```python
from build123d import *

# Parameters (mm, degrees)
SKETCH1_R           = 2.4
BOSS_EXTRUDE1_DEPTH = 2
SKETCH2_R           = 1.5
BOSS_EXTRUDE2_DEPTH = 5
FILLET1_R           = 0.5
CUT_EXTRUDE1_DEPTH  = 0.5


with BuildPart() as part:
    # Sketch1 → Boss-Extrude1 (new body)
    with BuildSketch(Plane(origin=(0, 0, 0), x_dir=(1, 0, 0), z_dir=(0, 1, 0))):
        with Locations(Location((0, 0, 0), (0, 0, 270))):
            Circle(SKETCH1_R)
    extrude(amount=BOSS_EXTRUDE1_DEPTH)

    # Sketch2 → Boss-Extrude2 (add)
    with BuildSketch(Plane(origin=(0, 2, 0), x_dir=(1, 0, 0), z_dir=(0, 1, 0))):
        with Locations(Location((0, 0, 0), (0, 0, 270))):
            Circle(SKETCH2_R)
    extrude(amount=BOSS_EXTRUDE2_DEPTH)

    # Fillet1
    fillet1_edges = [part.edges().sort_by_distance(p)[0] for p in [
        (0, 0, -2.4),
        (0, 2, -2.4),
    ]]
    fillet(fillet1_edges, radius=FILLET1_R)

    # Sketch3 → Cut-Extrude1 (cut)
    with BuildSketch(Plane.XZ):
        Polygon((0.5, 0.5), (1.5, 0.5), (1.5, -0.5), (0.5, -0.5), (0.5, -1.5), (-0.5, -1.5), (-0.5, -0.5), (-1.5, -0.5), (-1.5, 0.5), (-0.5, 0.5), (-0.5, 1.5), (0.5, 1.5), align=None)
    extrude(amount=-CUT_EXTRUDE1_DEPTH, mode=Mode.SUBTRACT)


solid = part.part
```
Verification items for the finished model (mm, model axes). A direction names the side the tool comes from. Coordinates: 2 decimals unless noted, no trailing zeros. Loops run counter-clockwise (first coordinate to the right, second up) from the corner with the lowest first, then second, coordinate; pieces in that order, holes last. Notation, with made-up numbers: (79, -17.5) -> (124, -17.5) arc R29 ccw to (124, 13.5) -> close; hole circle Ø1 at (55.5, 54). An arc over 180 degrees is marked (long way). Answer in a Markdown table with one row per item.
1) Section check C-C (y = 2.25). Record the cut outline in (x, z).
The answers:
| item | result |
|---|---|
| outline | circle Ø3 at (0, 0) |
2) Draft check along X on faces 3 (the face through (0, 7, 0)), 4 (the face through (0, 0.5, 0)), 5 (the face through (2.024, 0.993, 1.29)). Enter one of: released by +X, released by -X, zero draft, split by the parting line, or undercut.
The answers:
| item | result |
|---|---|
| face 3 | zero draft |
| face 4 | undercut |
| face 5 | split by the parting line |
3) Access from +Z, -Z, +X, -X, +Y, -Y to the whole of each face (thin tool, end or side, straight path). Record for faces 1 (the face through (0.45, 4.46, 1.43)), 2 (the face through (-1, 0, 1)).
The answers:
| item | result |
|---|---|
| face 1 | +Y |
| face 2 | +Z, -Z, +X, -X, -Y |
4) Section check A-A (x = 0). Record the cut outline in (y, z).
The answers:
| item | result |
|---|---|
| outline | (0, -1.9) arc R0.5 ccw to (0.5, -2.4) -> (1.5, -2.4) arc R0.5 ccw to (2, -1.9) -> (2, -1.5) -> (7, -1.5) -> (7, 1.5) -> (2, 1.5) -> (2, 1.9) arc R0.5 ccw to (1.5, 2.4) -> (0.5, 2.4) arc R0.5 ccw to (0, 1.9) -> (0, 1.5) -> (0.5, 1.5) -> (0.5, -1.5) -> (0, -1.5) -> close |
5) Scan lines: line 1 along Y through (x, z) = (-0.3, -1.05); line 2 along Y through (x, z) = (1.1, -1.6); line 3 along Z through (x, y) = (-0.25, 4.75). Record each from-to range of solid material in increasing order. Write a range as from..to.
The answers:
| item | result |
|---|---|
| line 1 | y = 0.5..7 |
| line 2 | y = 0..2 |
| line 3 | z = -1.48..1.48 |
6) Section check B-B (z = 0). Record the cut outline in (x, y), and give its area (3 significant figures).
The answers:
| item | result |
|---|---|
| outline | (-2.4, 0.5) arc R0.5 ccw to (-1.9, 0) -> (-1.5, 0) -> (-1.5, 0.5) -> (1.5, 0.5) -> (1.5, 0) -> (1.9, 0) arc R0.5 ccw to (2.4, 0.5) -> (2.4, 1.5) arc R0.5 ccw to (1.9, 2) -> (1.5, 2) -> (1.5, 7) -> (-1.5, 7) -> (-1.5, 2) -> (-1.9, 2) arc R0.5 ccw to (-2.4, 1.5) -> close |
| area | 22.9 mm2 |
7) Depth check by flat-ended pin: P1, Ø0.6, axis at y = 0.5, z = -1, coming from the -X side; P2, Ø1, axis at x = 1.5, y = 4.5, coming from the +Z side; P3, Ø0.6, axis at y = 0, z = 0, coming from the +X side. Enter the tip coordinate at first touch or a pass-through.
The answers:
| item | result |
|---|---|
| P1 | stops at x = -2.3 |
| P2 | stops at z = 1.12 |
| P3 | stops at x = 2.36 |
